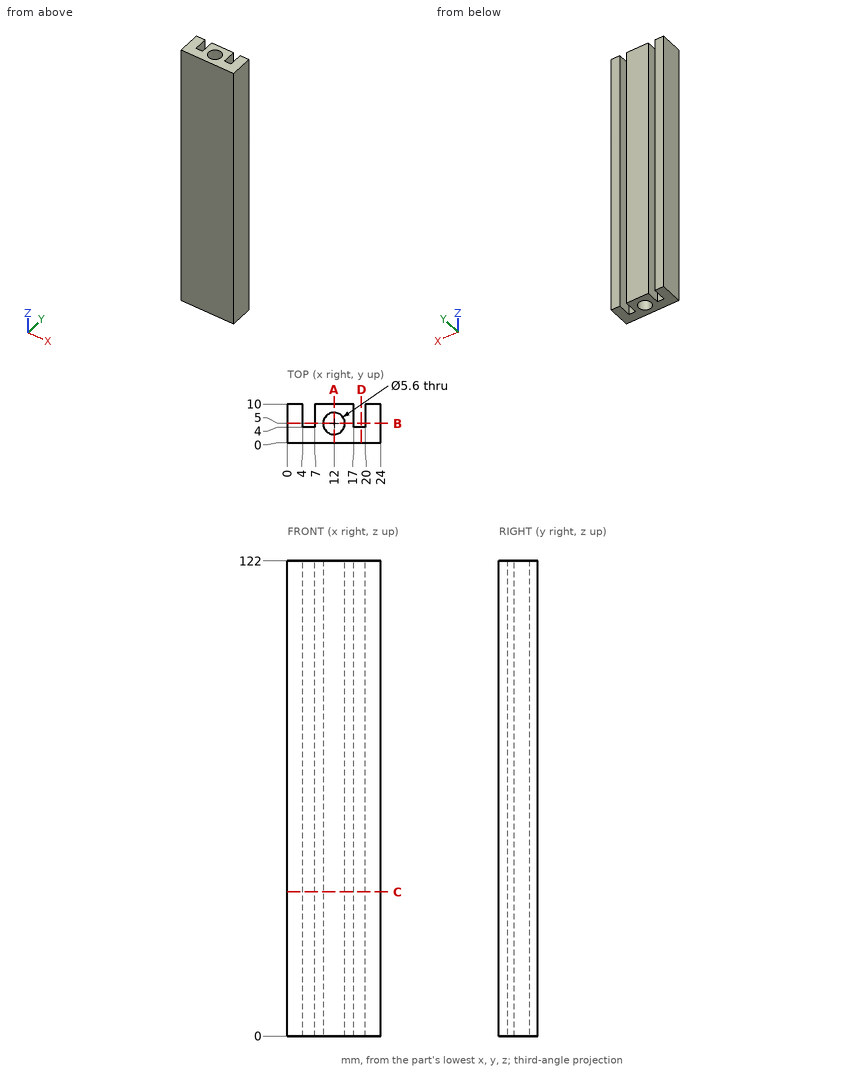
Answer from the drawing. Dimensions are ordinates in mm from the lowest x, y and z of the part. Give positions to 0.01 mm unless a question says otherwise; leave off trailing zeros. Write each loop counter-clockwise with the first axis right and the second up, starting at its lowest first coordinate (ties: lowest second). Pieces come first, ordered by that corner, then holes.
1) Find the intervals of material crossed by L1, parallel to Y at x = 12, z = 71.5; L2, parallel to X at y = 5.5, z = 40 (3 decimals); L3, parallel to X at y = 6.25, z = 26.5, in increasing order.
2) Section C-C (z = 37) is taken. Write down the section's boundary in (x, y).
3) Given P1, Ø0.9, axis at x = 18.5, z = 59, coming from the +Y side, flat-ended and moving along its own axis, determine where the tip first touches the part or whether it passes through.
4) Section B-B (y = 5) is taken. Write down the section's boundary in (x, z), and give its area (3 significant figures).
5) Section A-A (x = 12) is taken. Write down the section's boundary in (y, z).
6) Section D-D (x = 19) is taken. Write down the section's boundary in (y, z).
Response:
1. L1: y = 0 to 2.2, 7.8 to 10
1. L2: x = 0 to 4, 7 to 9.245, 14.755 to 17, 20 to 24
1. L3: x = 0 to 4, 7 to 9.49, 14.51 to 17, 20 to 24
2. outline: (0, 0) - (24, 0) - (24, 10) - (20, 10) - (20, 4) - (17, 4) - (17, 10) - (7, 10) - (7, 4) - (4, 4) - (4, 10) - (0, 10) - close; hole circle Ø5.6 at (12, 5)
3. P1: stops at y = 4
4. outline: (0, 0) - (4, 0) - (4, 122) - (0, 122) - close; (7, 0) - (9.2, 0) - (9.2, 122) - (7, 122) - close; (14.8, 0) - (17, 0) - (17, 122) - (14.8, 122) - close; (20, 0) - (24, 0) - (24, 122) - (20, 122) - close
4. area: 1,510 mm2
5. outline: (0, 0) - (2.2, 0) - (2.2, 122) - (0, 122) - close; (7.8, 0) - (10, 0) - (10, 122) - (7.8, 122) - close
6. outline: (0, 0) - (4, 0) - (4, 122) - (0, 122) - close
